Verification items for the finished model (mm, model axes). A direction names the side the tool comes from. Round coordinates to 2 decimals unless told otherwise and drop trailing zeros. Write each loop counter-clockwise with the first axis right and the second up, starting at its lowest first coordinate (ties: lowest second). Pieces come first, ordered by that corner, then holes. Notation, with made-up numbers: (-10.5, -33) - (5.5, -33) arc R19 cw to (5.5, 2) - close; hole circle Ø9 at (-27, 26.5). An arc over 180 degrees is marked (long way). Answer as a JSON object with one key per item and string values. Group by question number.
1) Thickness scan on line 1 (X direction, y = 0.1, z = -1); line 2 (Z direction, x = -72.5, y = 1.5) (1 decimal); line 3 (Z direction, x = -93.5, y = 1.45) (3 decimals). Record the ranges inside material, lowest first.
2) Section check D-D (x = -98). Enter the section's corners in (y, z) (3 decimals).
3) Go/stop test with flat-tipped pins: pin 1 Ø0.6 at (x, y) = (-71.5, 1) entering from +Z (3 decimals); pin 2 Ø1 at (y, z) = (1, -9.5) entering from +X. Record where each tip stops, or that it passes through.
4) Section check A-A (x = 7). Enter the section's corners in (y, z), then the cut area to 3 significant figures.
5) Set-up check for faces 1 (the flat face through (-36, 2, -10)), 2 (the flat face through (-80, 1, -0.375)): record each of +Z, -Z, +X, -X, +Y, -Y from which the full face is reachable in a straight line by a thin tool's end or side.
6) Mould release check, pull along Z, two halves, no side actions. Record for faces 3 (the flat face through (-36, 0, -10)), 4 (the flat face through (-96.17, 0.99, -12.37)), 5 (the cylindrical face through (-93.954, 0.986, -2.43)): +Z half, -Z half, draft (parallel to the pull), parting line (faces both ways), or undercut.
7) Section check C-C (x = -85.5). Enter the section's corners in (y, z) (3 decimals), then the cut area to 3 significant figures.
8) Section check B-B (y = 1.05). State how many separate pieces and enclosed holes the cut face has, then the cut area to 3 significant figures.
```python
from build123d import *

# Parameters (mm, degrees)
SKETCH1_R                = 1.25
SKETCH1_R_2              = 1.75
BOSS_EXTRUDE1_DEPTH      = 2
FILLET_1_R               = 1
SKETCH_1_R               = 1.25
CUT_EXTRUDE_1_DEPTH      = 1
CUT_EXTRUDE_1_DEPTH_BACK = 3


with BuildPart() as part:
    # Sketch1 → Boss-Extrude1 (new body)
    with BuildSketch(Plane(origin=(0, 0, 0), x_dir=(1, 0, 0), z_dir=(0, 1, 0))):
        with BuildLine():
            Line((-13.417150151, 22.383876488), (-69.977405348, 22.383876488))
            Line((-69.977405348, 22.383876488), (-86.593533576, 22.383876488))
            Line((-86.593533576, 22.383876488), (-107.641374678, 0.375))
            Line((-107.641374678, 0.375), (-53.661481565, 0.375))
            Line((-53.661481565, 0.375), (-53, 0))
            Line((-53, 0), (0, -10))
            Line((0, -10), (0, -3.5))
            ThreePointArc((0, -3.5), (-3.5, 0), (0, 3.5))
            Line((0, 3.5), (0, 10))
            ThreePointArc((0, 10), (6.493821579, 7.604622364), (9.876612161, 1.566056261))
            ThreePointArc((9.876612161, 1.566056261), (2.20319717, 16.421011896), (-13.417150151, 22.383876488))
        make_face()
        with Locations((-92.705183178, 2.375)):
            Circle(SKETCH1_R, mode=Mode.SUBTRACT)
        with Locations((-70.705183178, 2.375)):
            Circle(SKETCH1_R, mode=Mode.SUBTRACT)
        with Locations((-3.5, -6.062177826)):
            Circle(SKETCH1_R_2, mode=Mode.SUBTRACT)
        with Locations((-3.5, 6.062177826)):
            Circle(SKETCH1_R_2, mode=Mode.SUBTRACT)
        with BuildLine():
            ThreePointArc((10, 0), (9.951428515, 0.784062032), (9.876612161, 1.566056261))
            ThreePointArc((9.876612161, 1.566056261), (6.493821579, 7.604622364), (0, 10))
            Line((0, 10), (0, 3.5))
            ThreePointArc((0, 3.5), (2.474873734, 2.474873734), (3.5, 0))
            ThreePointArc((3.5, 0), (2.474873734, -2.474873734), (0, -3.5))
            Line((0, -3.5), (0, -10))
            ThreePointArc((0, -10), (7.071067812, -7.071067812), (10, 0))
        make_face()
        with Locations((7, 0)):
            Circle(SKETCH1_R_2, mode=Mode.SUBTRACT)
    extrude(amount=BOSS_EXTRUDE1_DEPTH)

    # Скругление1
    fillet_1_edges = [part.edges().sort_by_distance(p)[0] for p in [
        (-107.641374678, 1, -0.375),
    ]]
    fillet(fillet_1_edges, radius=FILLET_1_R)

    # Эскиз1 → Вырез-Вытянуть1 (cut, two sides)
    with BuildSketch(Plane(origin=(0, 2, 0), x_dir=(1, 0, 0), z_dir=(0, 1, 0))) as cut_extrude_1_sk:
        with Locations((-92.593533576, 10.375)):
            Circle(SKETCH_1_R)
        with Locations((-72.593533576, 10.375)):
            Circle(SKETCH_1_R)
        with Locations((-52.593533576, 10.375)):
            Circle(SKETCH_1_R)
    extrude(amount=CUT_EXTRUDE_1_DEPTH, mode=Mode.SUBTRACT)
    extrude(cut_extrude_1_sk.sketch, amount=-CUT_EXTRUDE_1_DEPTH_BACK, mode=Mode.SUBTRACT)


solid = part.part
```
Returned:
{
 "1": {"line 1": "-106.23 to -3.35, 3.35 to 5.56, 8.44 to 9.93", "line 2": "-22.4 to -11.6, -9.1 to -0.4", "line 3": "-15.162 to -11.236, -9.514 to -3.34, -1.41 to -0.375"},
 "2": {"outline": "(0, -10.457) - (2, -10.457) - (2, -0.375) - (0, -0.375) - close"},
 "3": {"pin 1": "z = -0.375", "pin 2": "x = 7.76"},
 "4": {"outline": "(0, -10.46) - (2, -10.46) - (2, -1.75) - (0, -1.75) - close; (0, 1.75) - (2, 1.75) - (2, 7.14) - (0, 7.14) - close", "area": "28.2 mm2"},
 "5": {"face 1": "+Z, -Z, +X, -X, +Y", "face 2": "+Z, -X, +Y, -Y"},
 "6": {"face 3": "draft", "face 4": "-Z half", "face 5": "undercut"},
 "7": {"outline": "(0, -22.384) - (2, -22.384) - (2, -0.375) - (0, -0.375) - close", "area": "44.0 mm2"},
 "8": {"separate pieces": "1", "enclosed holes": "9", "area": "2,510 mm2"}
}
